The model under review builds one solid part; all positions refer to its coordinate system, in mm. Face numbers are marked on the shaded views. Coordinates: 2 decimals unless noted, no trailing zeros. Order: outer loops, then holes, each group sorted by start corner. A loop starts at its lowest first (then second) coordinate and runs counter-clockwise, first axis right, second up. Notation, with made-up numbers: (-17.5, 78.5) -> (32.5, 78.5) arc R21 ccw to (32.5, 99.5) -> close; hole circle Ø7 at (-1, 57.5). An arc over 180 degrees is marked (long way). Put each result on its own line as item: value.
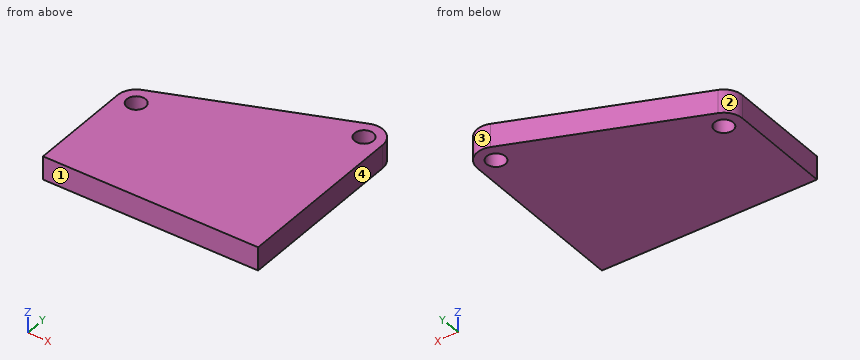
Autodesk Inventor part; units mm, degrees
ref_plane "YZ Plane" through (0, 0, 0) normal (1, 0, 0) x (0, 1, 0)
ref_plane "XZ Plane" through (0, 0, 0) normal (0, 1, 0) x (-1, 0, 0)
ref_plane "XY Plane" through (0, 0, 0) normal (0, 0, 1) x (1, 0, 0)
sketch "スケッチ1" plane through (0, 0, 0) normal (0, 0, 1) x (1, 0, 0)
  line L0 (0, 0) -> (38, 14.94) construction
  line L1 (36.5364, 18.6626) -> (-1.4636, 3.7226)
  line L2 (-4, 0) -> (-4, -22.2053)
  line L3 (-4, -22.2053) -> (42, -22.2053)
  line L4 (42, -22.2053) -> (42, 14.94)
  arc A0 (-1.4636, 3.7226) -> (-4, 0) centre (0, 0) ccw
  arc A1 (42, 14.94) -> (36.5364, 18.6626) centre (38, 14.94) ccw
  dimension "d0" = 38
  dimension "d1" = 14.94
  dimension "d2" = 4
extrude "押し出し1" add sketch "スケッチ1" along normal blind 5
hole "穴1" at (0, 0, 0) at (38, 14.94, 0) direction (0, 0, 1) diameter 4 end through all
properties part number "COXA_ROLL_COUPLER_BACK"
Item 1: For pin 1 Ø1.5 at (x, z) = (1.5, 1.5) entering from +Y, flat-tipped, find the tip position at first contact; note if it passes through.
Answers below:
pin 1: y = 5.18
Item 2: Consider section D-D on y = 9. Write out the cut boundary in (x, z), and give its area (3 significant figures).
Answers below:
outline: (11.96, 0) -> (42, 0) -> (42, 5) -> (11.96, 5) -> close
area: 150 mm^2
Item 3: Consider section B-B on z = 1.1. Write out the cut boundary in (x, y), and give its area (3 significant figures).
Answers below:
outline: (-4, -22.21) -> (42, -22.21) -> (42, 14.94) arc R4 ccw to (36.54, 18.66) -> (-1.46, 3.72) arc R4 ccw to (-4, 0) -> close; hole circle Ø4 at (0, 0); hole circle Ø4 at (38, 14.94)
area: 1,530 mm^2
Item 4: Consider section A-A on x = 38. Write out the cut boundary in (y, z).
Answers below:
outline: (-22.21, 0) -> (12.94, 0) -> (12.94, 5) -> (-22.21, 5) -> close; (16.94, 0) -> (18.94, 0) -> (18.94, 5) -> (16.94, 5) -> close
Item 5: Consider section C-C on x = 0. Write out the cut boundary in (y, z), and give its area (3 significant figures).
Answers below:
outline: (-22.21, 0) -> (-2, 0) -> (-2, 5) -> (-22.21, 5) -> close; (2, 0) -> (4.3, 0) -> (4.3, 5) -> (2, 5) -> close
area: 113 mm^2
Item 6: For line 1 (X direction, y = 0, z = 1.55); line 2 (Y direction, x = 38, z = 2.8); line 3 (Y direction, x = 22, z = 0.45), list the stretches that pass through material, from the lowest coordinate up. Write a range as from..to.
Answers below:
line 1: -4..-2, 2..42
line 2: -22.21..12.94, 16.94..18.94
line 3: -22.21..12.95
Item 7: Mouldability with a two-part tool opening along X and no side actions: class the marked faces 1, 2, 3 and 4 as +X half, -X half, draft (parallel to the pull), parting line (faces both ways), or undercut.
Answers below:
face 1: draft
face 2: -X half
face 3: parting line
face 4: +X half
